Part model, mm, in its own coordinate system. A direction names the side the tool comes from. Round coordinates to 2 decimals unless told otherwise and drop trailing zeros. Order: outer loops, then holes, each group sorted by start corner. A loop starts at its lowest first (then second) coordinate and runs counter-clockwise, first axis right, second up. Notation, with made-up numbers: M 79,48.5 L 119,48.5 A19 ccw 119,81.5 Z; hole C -25.75,-19.75 d9. An arc over 180 degrees is marked long. One line per question, with ' | ' between items.
from build123d import *

# Parameters (mm, degrees)
SKETCH1_W           = 126
SKETCH1_H           = 71
BOSS_EXTRUDE1_DEPTH = 31
SKETCH2_W           = 120.6
SKETCH2_H           = 66
CUT_EXTRUDE1_DEPTH  = 22
CUT_EXTRUDE2_REACH  = 136.526
SKETCH3_W           = 33
SKETCH3_H           = 6
FILLET1_R           = 4.8
BOSS_EXTRUDE2_DEPTH = 2.5
CUT_EXTRUDE3_DEPTH  = 88.916153237
SKETCH6_R           = 1.5
CUT_EXTRUDE4_DEPTH  = 88.916153237
FILLET2_R           = 2
FILLET3_R           = 1
BOSS_EXTRUDE3_DEPTH = 4.7
BOSS_EXTRUDE4_START = 5.3
BOSS_EXTRUDE4_DEPTH = 5.3
CUT_EXTRUDE5_DEPTH  = 60.5
CUT_EXTRUDE6_REACH  = 100.093
BOSS_EXTRUDE5_DEPTH = 5.62751
BOSS_EXTRUDE6_DEPTH = 5.62751
BOSS_EXTRUDE7_DEPTH = 5.62751


with BuildPart() as part:
    # Sketch1 → Boss-Extrude1 (new body)
    with BuildSketch(Plane(origin=(0, 0, 0), x_dir=(1, 0, 0), z_dir=(0, 1, 0))):
        Rectangle(SKETCH1_W, SKETCH1_H)
    extrude(amount=BOSS_EXTRUDE1_DEPTH)

    # Sketch2 → Cut-Extrude1 (cut)
    with BuildSketch(Plane.XZ):
        with Locations((-0.2, 0)):
            Rectangle(SKETCH2_W, SKETCH2_H)
    extrude(amount=-CUT_EXTRUDE1_DEPTH, mode=Mode.SUBTRACT)

    # Sketch3 → Cut-Extrude2 (cut, up to next)
    with BuildSketch(Plane(origin=(63, 0, 0), x_dir=(0, 0, -1), z_dir=(1, 0, 0)), mode=Mode.PRIVATE) as cut_extrude2_sk1:
        with Locations((0.5, 3)):
            Rectangle(SKETCH3_W, SKETCH3_H)
    cut_extrude2_tool1 = extrude(cut_extrude2_sk1.sketch, amount=-CUT_EXTRUDE2_REACH, mode=Mode.PRIVATE) & part.part
    add(cut_extrude2_tool1.solids().sort_by_distance((63, 3, -0.5))[0], mode=Mode.SUBTRACT)

    # Fillet1
    fillet1_edges = [part.edges().sort_by_distance(p)[0] for p in [
        (61.55, 6, -17),
        (61.55, 6, 16),
    ]]
    fillet(fillet1_edges, radius=FILLET1_R)

    # Sketch4 → Boss-Extrude2 (add)
    with BuildSketch(Plane.ZY.offset(63)):
        Polygon((-32.6, 0), (-32.6, -19), (5, -19), (5, -6), (32.4, -6), (32.4, 0), align=None)
    extrude(amount=-BOSS_EXTRUDE2_DEPTH)

    # Sketch5 → Cut-Extrude3 (cut, through all)
    with BuildSketch(Plane(origin=(0, 31, 0), x_dir=(1, 0, 0), z_dir=(0, 1, 0))):
        with BuildLine():
            Line((3.5, 4.898979486), (3.5, 7.937253933))
            ThreePointArc((3.5, 7.937253933), (8.156854249, 5.656854249), (10.437253933, 1))
            Line((10.437253933, 1), (7.398979486, 1))
            ThreePointArc((7.398979486, 1), (6.035533906, 3.535533906), (3.5, 4.898979486))
        make_face()
        with BuildLine():
            Line((1.5, -4.898979486), (1.5, -7.937253933))
            ThreePointArc((1.5, -7.937253933), (-3.156854249, -5.656854249), (-5.437253933, -1))
            Line((-5.437253933, -1), (-2.398979486, -1))
            ThreePointArc((-2.398979486, -1), (-1.035533906, -3.535533906), (1.5, -4.898979486))
        make_face()
        with BuildLine():
            Line((7.398979486, -1), (10.437253933, -1))
            ThreePointArc((10.437253933, -1), (8.156854249, -5.656854249), (3.5, -7.937253933))
            Line((3.5, -7.937253933), (3.5, -4.898979486))
            ThreePointArc((3.5, -4.898979486), (6.035533906, -3.535533906), (7.398979486, -1))
        make_face()
        with BuildLine():
            Line((-2.398979486, 1), (-5.437253933, 1))
            ThreePointArc((-5.437253933, 1), (-3.156854249, 5.656854249), (1.5, 7.937253933))
            Line((1.5, 7.937253933), (1.5, 4.898979486))
            ThreePointArc((1.5, 4.898979486), (-1.035533906, 3.535533906), (-2.398979486, 1))
        make_face()
        with BuildLine():
            Line((1.5, 10.95445115), (1.5, 13.964240044))
            ThreePointArc((1.5, 13.964240044), (-7.399494937, 9.899494937), (-11.464240044, 1))
            Line((-11.464240044, 1), (-8.45445115, 1))
            ThreePointArc((-8.45445115, 1), (-5.278174593, 7.778174593), (1.5, 10.95445115))
        make_face()
        with BuildLine():
            Line((1.5, 16.970562748), (1.5, 19.974984355))
            ThreePointArc((1.5, 19.974984355), (-11.642135624, 14.142135624), (-17.474984355, 1))
            Line((-17.474984355, 1), (-14.470562748, 1))
            ThreePointArc((-14.470562748, 1), (-9.52081528, 12.02081528), (1.5, 16.970562748))
        make_face()
        with BuildLine():
            Line((3.5, 16.970562748), (3.5, 19.974984355))
            ThreePointArc((3.5, 19.974984355), (16.642135624, 14.142135624), (22.474984355, 1))
            Line((22.474984355, 1), (19.470562748, 1))
            ThreePointArc((19.470562748, 1), (14.52081528, 12.02081528), (3.5, 16.970562748))
        make_face()
        with BuildLine():
            Line((3.5, 10.95445115), (3.5, 13.964240044))
            ThreePointArc((3.5, 13.964240044), (12.399494937, 9.899494937), (16.464240044, 1))
            Line((16.464240044, 1), (13.45445115, 1))
            ThreePointArc((13.45445115, 1), (10.278174593, 7.778174593), (3.5, 10.95445115))
        make_face()
        with BuildLine():
            Line((-8.45445115, -1), (-11.464240044, -1))
            ThreePointArc((-11.464240044, -1), (-7.399494937, -9.899494937), (1.5, -13.964240044))
            Line((1.5, -13.964240044), (1.5, -10.95445115))
            ThreePointArc((1.5, -10.95445115), (-5.278174593, -7.778174593), (-8.45445115, -1))
        make_face()
        with BuildLine():
            Line((-14.470562748, -1), (-17.474984355, -1))
            ThreePointArc((-17.474984355, -1), (-11.642135624, -14.142135624), (1.5, -19.974984355))
            Line((1.5, -19.974984355), (1.5, -16.970562748))
            ThreePointArc((1.5, -16.970562748), (-9.52081528, -12.02081528), (-14.470562748, -1))
        make_face()
        with BuildLine():
            Line((3.5, -10.95445115), (3.5, -13.964240044))
            ThreePointArc((3.5, -13.964240044), (12.399494937, -9.899494937), (16.464240044, -1))
            Line((16.464240044, -1), (13.45445115, -1))
            ThreePointArc((13.45445115, -1), (10.278174593, -7.778174593), (3.5, -10.95445115))
        make_face()
        with BuildLine():
            Line((3.5, -16.970562748), (3.5, -19.974984355))
            ThreePointArc((3.5, -19.974984355), (16.642135624, -14.142135624), (22.474984355, -1))
            Line((22.474984355, -1), (19.470562748, -1))
            ThreePointArc((19.470562748, -1), (14.52081528, -12.02081528), (3.5, -16.970562748))
        make_face()
    extrude(amount=-CUT_EXTRUDE3_DEPTH, mode=Mode.SUBTRACT)

    # Sketch6 → Cut-Extrude4 (cut, through all)
    with BuildSketch(Plane(origin=(0, 31, 0), x_dir=(1, 0, 0), z_dir=(0, 1, 0))):
        with Locations(Location((-13.5, 16, 0), (0, 0, 270))):
            Circle(SKETCH6_R)
        with Locations(Location((18.5, 16, 0), (0, 0, 270))):
            Circle(SKETCH6_R)
        with Locations(Location((18.5, -16, 0), (0, 0, 270))):
            Circle(SKETCH6_R)
        with Locations(Location((-13.5, -16, 0), (0, 0, 270))):
            Circle(SKETCH6_R)
    extrude(amount=-CUT_EXTRUDE4_DEPTH, mode=Mode.SUBTRACT)

    # Fillet2
    fillet2_edges = [part.edges().sort_by_distance(p)[0] for p in [
        (-63, 15.5, 35.5),
        (-63, 15.5, -35.5),
        (63, 15.5, -35.5),
        (63, 15.5, 35.5),
    ]]
    fillet(fillet2_edges, radius=FILLET2_R)

    # Fillet3
    fillet3_edges = [part.edges().sort_by_distance(p)[0] for p in [
        (0, 31, 35.5),
        (-63, 31, 0),
        (63, 31, 0),
        (0, 31, -35.5),
        (62.414213562, 31, 34.914213562),
        (62.414213562, 31, -34.914213562),
        (-62.414213562, 31, -34.914213562),
        (-62.414213562, 31, 34.914213562),
    ]]
    fillet(fillet3_edges, radius=FILLET3_R)

    # Sketch7 → Boss-Extrude3 (add)
    with BuildSketch(Plane.XZ):
        with BuildLine():
            Line((-57.313755, 32.51305), (-57.313755, 33))
            Line((-57.313755, 33), (-51.686245, 33))
            Line((-51.686245, 33), (-51.686245, 32.51305))
            ThreePointArc((-51.686245, 32.51305), (-54.5, 29.699295), (-57.313755, 32.51305))
        make_face()
        with BuildLine():
            Line((-57.313755, -32.51305), (-57.313755, -33))
            Line((-57.313755, -33), (-51.686245, -33))
            Line((-51.686245, -33), (-51.686245, -32.51305))
            ThreePointArc((-51.686245, -32.51305), (-54.5, -29.699295), (-57.313755, -32.51305))
        make_face()
        with BuildLine():
            Line((60.01305, -25.813755), (60.1, -25.813755))
            Line((60.1, -25.813755), (60.1, -20.186245))
            Line((60.1, -20.186245), (60.01305, -20.186245))
            ThreePointArc((60.01305, -20.186245), (57.199295, -23), (60.01305, -25.813755))
        make_face()
        with BuildLine():
            Line((60.01305, 25.813755), (60.1, 25.813755))
            Line((60.1, 25.813755), (60.1, 20.186245))
            Line((60.1, 20.186245), (60.01305, 20.186245))
            ThreePointArc((60.01305, 20.186245), (57.199295, 23), (60.01305, 25.813755))
        make_face()
    extrude(amount=-BOSS_EXTRUDE3_DEPTH)

    # Sketch8 → Boss-Extrude4 (add)
    with BuildSketch(Plane.XZ.offset(BOSS_EXTRUDE4_START)):
        with BuildLine():
            Line((-57.313755, 33), (-57.313755, 32.51305))
            ThreePointArc((-57.313755, 32.51305), (-54.5, 29.699295), (-51.686245, 32.51305))
            Line((-51.686245, 32.51305), (-51.686245, 33))
            Line((-51.686245, 33), (-57.313755, 33))
        make_face()
        with BuildLine():
            Line((-57.313755, -32.51305), (-57.313755, -33))
            Line((-57.313755, -33), (-51.686245, -33))
            Line((-51.686245, -33), (-51.686245, -32.51305))
            ThreePointArc((-51.686245, -32.51305), (-54.5, -29.699295), (-57.313755, -32.51305))
        make_face()
        with BuildLine():
            Line((60.01305, -25.813755), (60.1, -25.813755))
            Line((60.1, -25.813755), (60.1, -20.186245))
            Line((60.1, -20.186245), (60.01305, -20.186245))
            ThreePointArc((60.01305, -20.186245), (57.199295, -23), (60.01305, -25.813755))
        make_face()
        with BuildLine():
            Line((60.01305, 20.186245), (60.1, 20.186245))
            Line((60.1, 20.186245), (60.1, 25.813755))
            Line((60.1, 25.813755), (60.01305, 25.813755))
            ThreePointArc((60.01305, 25.813755), (57.199295, 23), (60.01305, 20.186245))
        make_face()
    extrude(amount=-BOSS_EXTRUDE4_DEPTH)

    # Sketch9 → Cut-Extrude5 (cut)
    with BuildSketch(Plane(origin=(0, 0, 0), x_dir=(0, 0, -1), z_dir=(1, 0, 0))):
        Polygon((-33, 4.7), (-29.699295, 1.399295), (-29.699295, 4.7), align=None)
        Polygon((33, 4.7), (29.699295, 1.399295), (29.699295, 4.7), align=None)
    extrude(amount=-CUT_EXTRUDE5_DEPTH, mode=Mode.SUBTRACT)

    # Cut-Extrude6: up to this face of the body (flat: up to its plane)
    cut_extrude6_end = Plane(part.part.faces().sort_by_distance((0.346757949, 11.087098642, 33))[0])
    # Sketch10 → Cut-Extrude6 (cut, up to the picked face)
    with BuildSketch(Plane.XY.offset(-33), mode=Mode.PRIVATE) as cut_extrude6_sk1:
        Polygon((60.1, 4.7), (57.199295, 1.799295), (57.199295, 4.7), align=None)
    cut_extrude6_tool1 = split(extrude(cut_extrude6_sk1.sketch, amount=CUT_EXTRUDE6_REACH, mode=Mode.PRIVATE), bisect_by=cut_extrude6_end, keep=Keep.BOTH, mode=Mode.PRIVATE)
    add(cut_extrude6_tool1.solids().sort_by(Axis((58.166197, 3.733098, -33), (0, 0, 1)))[0], mode=Mode.SUBTRACT)

    # Sketch11 → Boss-Extrude5 (add)
    with BuildSketch(Plane.XY.offset(25.813755)):
        Polygon((60.1, -3.3), (62.1, -3.3), (62.1, -3.5), (60.3, -5.3), (60.1, -5.3), align=None)
    extrude(amount=-BOSS_EXTRUDE5_DEPTH)

    # Sketch12 → Boss-Extrude6 (add)
    with BuildSketch(Plane.XY.offset(-20.186245)):
        Polygon((60.1, -3.3), (62.1, -3.3), (62.1, -3.5), (60.3, -5.3), (60.1, -5.3), align=None)
    extrude(amount=-BOSS_EXTRUDE6_DEPTH)

    # Sketch13 → Boss-Extrude7 (add)
    with BuildSketch(Plane(origin=(-51.686245, 0, 0), x_dir=(0, 0, -1), z_dir=(1, 0, 0))):
        Polygon((-33, -3.3), (-35, -3.3), (-35, -3.5), (-33.2, -5.3), (-33, -5.3), align=None)
        Polygon((33, -5.3), (33.2, -5.3), (35, -3.5), (35, -3.3), (33, -3.3), align=None)
    extrude(amount=-BOSS_EXTRUDE7_DEPTH)


solid = part.part
1) Drop flat-ended pins along their axis: pin 1 (2 mm diameter, centred on x = -62, z = 20, fed in from -Y); pin 2 (1 mm diameter, centred on x = -29.5, z = -19, fed in from -Y); pin 3 (12 mm diameter, centred on x = 22, y = -3.5, fed in from -Z); pin 4 (1 mm diameter, centred on y = -10, z = 0.5, fed in from +X). Give the stop position or say it passes through.
The answers:
pin 1: stops at y = -6 | pin 2: stops at y = 22 | pin 3: stops at z = -35.5 | pin 4: stops at x = -60.5
2) Saw through at D-D (z = -2.5). Give the number of separate pieces and of enclosed holes in the cut face, plus the area to 3 significant figures.
The answers:
separate pieces: 7 | enclosed holes: 0 | area: 1,110 mm²
3) Saw through at C-C (z = -23). List the corners of the cut face in (x, y).
The answers:
outline: M -63,-19 L -60.5,-19 L -60.5,22 L 60.1,22 L 60.1,4.7 L 57.2,1.8 L 57.2,-5.3 L 60.3,-5.3 L 62.1,-3.5 L 62.1,-3.3 L 60.1,-3.3 L 60.1,0 L 63,0 L 63,30 A1 ccw 62,31 L -62,31 A1 ccw -63,30 Z
4) Which spindle directions (+Z, -Z, +X, -X, +Y, -Y) get a long thin tool onto all of the face, cutting with end or side? Do faces 3 (the face through (57.2, -1.5, -22.9)), 4 (the face through (61.53, 4.56, -15.63)), 5 (the face through (14.64, 26.56, -11.9)). Say none if no direction does.
The answers:
face 3: -Y | face 4: +X, -Y | face 5: +Y, -Y
5) Two-plate mould, pull along X, no slides. Class faces 1 (the face through (-51.686, -1.8, 32.8)), 2 (the face through (-62, -19, -14)): released by +X, released by -X, zero draft, split by the parting line, or undercut.
The answers:
face 1: undercut | face 2: zero draft
6) Saw through at A-A (y = 12). List the corners of the cut face in (x, z), plus the area to 3 significant figures.
The answers:
outline: M -63,-33.5 A2 ccw -61,-35.5 L 61,-35.5 A2 ccw 63,-33.5 L 63,33.5 A2 ccw 61,35.5 L -61,35.5 A2 ccw -63,33.5 Z; hole M -60.5,-33 L 60.1,-33 L 60.1,33 L -60.5,33 Z | area: 983 mm²
7) Saw through at B-B (x = 29.5). List the corners of the cut face in (y, z).
The answers:
outline: M 0,-35.5 L 30,-35.5 A1 ccw 31,-34.5 L 31,34.5 A1 ccw 30,35.5 L 0,35.5 L 0,33 L 22,33 L 22,-33 L 0,-33 Z
8) Probe line 1 (Z direction, x = -39, y = 17); line 2 (X direction, y = 11, z = -11.5); line 3 (Y direction, x = -30, z = 15). List the from-to ranges inside material, lowest first. Write a range as [from, to].
The answers:
line 1: z = [-35.5, -33], [33, 35.5] | line 2: x = [-63, -60.5], [60.1, 63] | line 3: y = [22, 31]
